Verification items for this drawing (mm, ordinates from the low corner). Round coordinates to 2 decimals unless told otherwise and drop trailing zeros. Order: outer loops, then holes, each group sorted by start corner. A loop starts at its lowest first (then second) coordinate and runs counter-clockwise, first axis right, second up. Notation, with made-up numbers: (85.5, 68.25) -> (97.5, 68.25) arc R11 ccw to (97.5, 78.25) -> close; hole circle Ø7 at (-38.75, 8.25). An arc over 180 degrees is marked (long way). Answer in a Markdown table with one row per item. Add a question column.
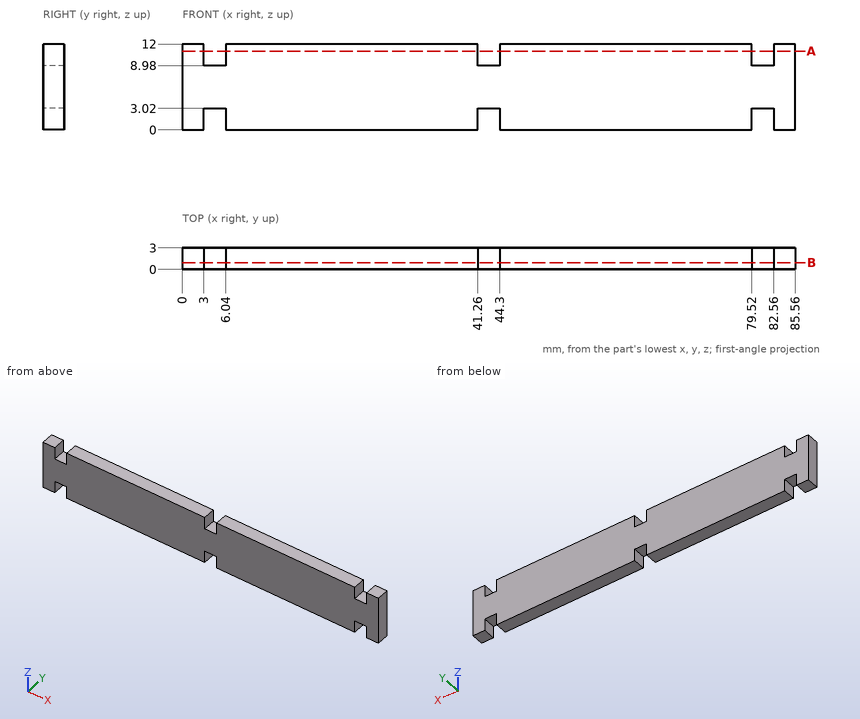
1) Cross-section at A-A, the plane z = 11. Record the boundary of the cut face in (x, y), and give its area (3 significant figures).
2) Cross-section at B-B, the plane y = 0.95. Record the boundary of the cut face in (x, z), and give its area (3 significant figures).
3) Thickness scan on L1, parallel to X at y = 2.25, z = 2; L2, parallel to Z at x = 41.5, y = 2.15. Record the ranges inside material, lowest first. Write a range as [from, to].
4) Depth check by flat-ended pin: P1, Ø1.5, axis at x = 4.5, y = 1.5, coming from the -Z side. Enter the tip coordinate at first touch or a pass-through.
Results below:
| question | item | result |
|---|---|---|
| 1 | outline | (0, 0) -> (3, 0) -> (3, 3) -> (0, 3) -> close; (6.04, 0) -> (41.26, 0) -> (41.26, 3) -> (6.04, 3) -> close; (44.3, 0) -> (79.52, 0) -> (79.52, 3) -> (44.3, 3) -> close; (82.56, 0) -> (85.56, 0) -> (85.56, 3) -> (82.56, 3) -> close |
| 1 | area | 229 mm² |
| 2 | outline | (0, 0) -> (3, 0) -> (3, 3.02) -> (6.04, 3.02) -> (6.04, 0) -> (41.26, 0) -> (41.26, 3.02) -> (44.3, 3.02) -> (44.3, 0) -> (79.52, 0) -> (79.52, 3.02) -> (82.56, 3.02) -> (82.56, 0) -> (85.56, 0) -> (85.56, 12) -> (82.56, 12) -> (82.56, 8.98) -> (79.52, 8.98) -> (79.52, 12) -> (44.3, 12) -> (44.3, 8.98) -> (41.26, 8.98) -> (41.26, 12) -> (6.04, 12) -> (6.04, 8.98) -> (3, 8.98) -> (3, 12) -> (0, 12) -> close |
| 2 | area | 972 mm² |
| 3 | L1 | [0, 3], [6.04, 41.26], [44.3, 79.52], [82.56, 85.56] |
| 3 | L2 | [3.02, 8.98] |
| 4 | P1 | z = 3.02 |
